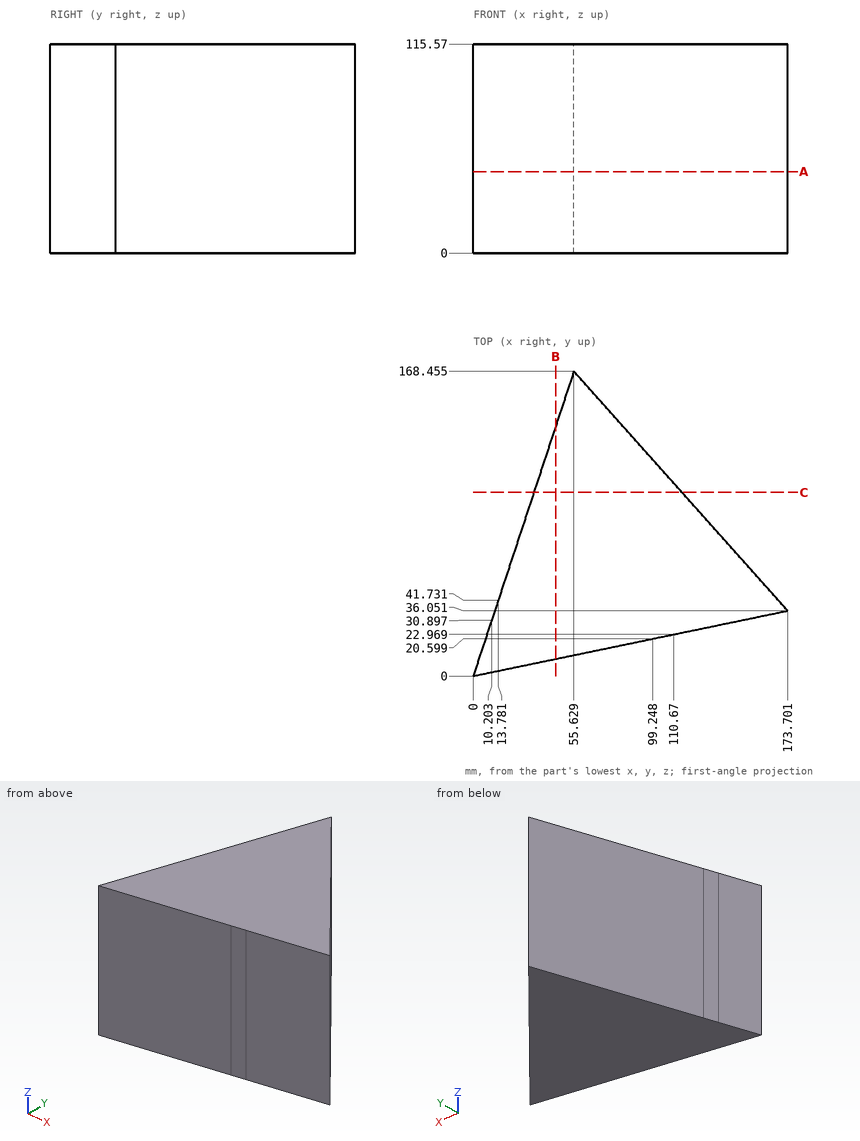
Drawing for the job (mm, zero at the part's lowest x, y, z). Round coordinates to 2 decimals unless told otherwise and drop trailing zeros. Write each loop counter-clockwise with the first axis right and the second up, starting at its lowest first coordinate (ties: lowest second). Pieces come first, ordered by that corner, then holes. Notation, with made-up numbers: (-25, -37.5) - (23, -37.5) arc R23 ccw to (23, -3.5) - close; hole circle Ø8 at (7.25, 22). An arc over 180 degrees is marked (long way). Write item = value, one per line. Start each with the question number.
Q1. Drop flat-ended pins along their axis: pin 1 (12 mm diameter, centred on y = 135, z = 94.5, fed in from -X); pin 2 (1.5 mm diameter, centred on y = 52.5, z = 41.5, fed in from +X); pin 3 (8 mm diameter, centred on x = 108, z = 61, fed in from -Y) (1 decimal); pin 4 (6 mm diameter, centred on x = 82.5, y = 146, fed in from +Z). Give the stop position or say it passes through.
Q2. Band-saw the part on B-B (x = 45.5). Give the cut face in (y, z).
Q3. Band-saw the part on A-A (z = 45). Give the cut face in (x, y) (1 decimal), then the cut area to 3 significant figures.
Q4. Band-saw the part on C-C (y = 101.5). Give the cut face in (x, z), then the cut area to 3 significant figures.
Q5. Probe L1, parallel to Y at x = 137, z = 12 (1 decimal); L2, parallel to X at y = 99, z = 59 (1 decimal); L3, parallel to Y at x = 84, z = 35 (1 decimal). List the from-to ranges inside material, lowest first. Write a range as from..to.
Answers below:
q1.pin_1 = 42.6
q1.pin_2 = 159.7
q1.pin_3 = 21.6
q1.pin_4 = through
q2.outline = (9.44, 0) - (137.78, 0) - (137.78, 115.57) - (9.44, 115.57) - close
q3.outline = (0, 0) - (173.7, 36.1) - (55.6, 168.5) - close
q3.area = 13,600 mm2
q4.outline = (33.52, 0) - (115.34, 0) - (115.34, 115.57) - (33.52, 115.57) - close
q4.area = 9,460 mm2
q5.L1 = 28.4..77.2
q5.L2 = 32.7..117.6
q5.L3 = 17.4..136.6
